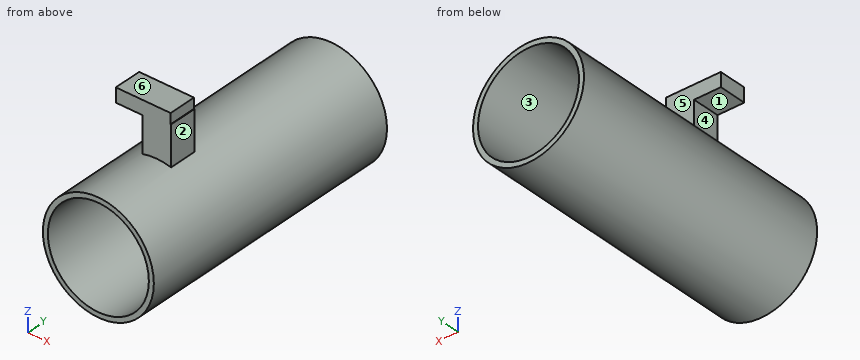
from build123d import *

# Parameters (mm, degrees)
F0_R     = 5.077075
F1_DEPTH = 25.4
F2_R     = 4.621365
F3_DEPTH = 25.4
F5_W     = 2.610316
F5_H     = 3.654443
F6_DEPTH = 2.54
F7_W     = 5.013653
F7_H     = 1.290941
F8_DEPTH = 2.54


with BuildPart() as f1:
    # F0 (on Front) → F1 (new body)
    with BuildSketch(Plane.XZ):
        Circle(F0_R)
    extrude(amount=F1_DEPTH)

    # F2 (on face) → F3 (cut)
    with BuildSketch(Plane.XZ.offset(25.4)):
        Circle(F2_R)
    extrude(amount=-F3_DEPTH, mode=Mode.SUBTRACT)

    # F5 (on offset) → F6 (join)
    with BuildSketch(Plane.XZ.offset(19.05)):
        with Locations((0.015271, 6.700735)):
            Rectangle(F5_W, F5_H)
    extrude(amount=-F6_DEPTH)

    # F7 (on offset) → F8 (join)
    with BuildSketch(Plane.XZ.offset(19.05)):
        with Locations((-1.230061, 8.832033)):
            Rectangle(F7_W, F7_H)
    extrude(amount=-F8_DEPTH)


solid = f1.part
Design review of the part built by this model. Coordinates are the model's own, in mm. Face numbers are marked on the shaded views. A direction names the side the tool comes from. Coordinates: 2 decimals unless noted, no trailing zeros. Loops run counter-clockwise (first coordinate to the right, second up) from the corner with the lowest first, then second, coordinate; pieces in that order, holes last.
Item 1: Add section C-C (x = -3). Write out the cut boundary in (y, z).
Completed:
outline: (-25.4, -4.1) - (0, -4.1) - (0, -3.52) - (-25.4, -3.52) - close; (-25.4, 3.52) - (0, 3.52) - (0, 4.1) - (-25.4, 4.1) - close; (-19.05, 8.19) - (-16.51, 8.19) - (-16.51, 9.48) - (-19.05, 9.48) - close
Item 2: Add section D-D (y = -10). Write out the cut boundary in (x, z).
Completed:
outline: circle Ø10.15 at (0, 0); hole circle Ø9.24 at (0, 0)
Item 3: Add section B-B (z = 0). Write out the cut boundary in (x, y).
Completed:
outline: (-5.08, -25.4) - (-4.62, -25.4) - (-4.62, 0) - (-5.08, 0) - close; (4.62, -25.4) - (5.08, -25.4) - (5.08, 0) - (4.62, 0) - close
Item 4: For the marked faces 1 and 2, list the 3-axis set-ups (+Z, -Z, +X, -X, +Y, -Y) from which the entire face can be reached by the end or side of a thin tool; tool diameter is ignored.
Completed:
face 1: -X, +Y, -Y
face 2: +Z, +X, +Y, -Y
Item 5: Clearance check with flat-ended pins moving along their axes: pin 1 (6 mm diameter, centred on y = -18.5, z = 1.5, fed in from +X); pin 2 (1.4 mm diameter, centred on x = 0, z = 7, fed in from +Y); pin 3 (2 mm diameter, centred on y = -18, z = 6.5, fed in from +X); pin 4 (1.2 mm diameter, centred on x = -2, y = -18, fed in from -Z). State where each tip first meets the part, or that it passes through.
Completed:
pin 1: stops at x = 5.08
pin 2: stops at y = -16.51
pin 3: stops at x = 1.32
pin 4: stops at z = -4.88
Item 6: Wall thickness on L1, parallel to Z at x = 0, y = -5.5; L2, parallel to X at y = -3.75, z = -2.5; L3, parallel to Z at x = 0, y = -17: over which ranges is each line inside the solid? List them lowest first.
Completed:
L1: z = -5.08 to -4.62, 4.62 to 5.08
L2: x = -4.42 to -3.89, 3.89 to 4.42
L3: z = -5.08 to -4.62, 4.62 to 9.48
Item 7: Add section A-A (x = 0). Write out the cut boundary in (y, z).
Completed:
outline: (-25.4, -5.08) - (0, -5.08) - (0, -4.62) - (-25.4, -4.62) - close; (-25.4, 4.62) - (0, 4.62) - (0, 5.08) - (-16.51, 5.08) - (-16.51, 9.48) - (-19.05, 9.48) - (-19.05, 5.08) - (-25.4, 5.08) - close
Item 8: Draft analysis for pull direction Z (two halves, no side actions). For the marked faces 3, 4, 5 and 6, state which applies: pulls with the +Z half, pulls with the -Z half, needs draft (parallel to the pull), parting line crosses it, or undercut.
Completed:
face 3: undercut
face 4: undercut
face 5: needs draft
face 6: pulls with the +Z half
